Source: CAD feature listing. Evaluate the final solid. Frame: model axes, mm. A direction names the side the tool comes from. Coordinates: 2 decimals unless noted, no trailing zeros. Write each loop counter-clockwise with the first axis right and the second up, starting at its lowest first coordinate (ties: lowest second). Pieces come first, ordered by that corner, then holes. Notation, with made-up numbers: M 4.5,-22.75 L 43.5,-22.75 A16 cw 43.5,-18.75 Z; hole C -14,-15 d5. An arc over 180 degrees is marked long. Answer as CSV lines item,"result". Start each with the question number.
1. Mould query, pull axis Z, two halves, no side actions, for faces 1 (the face through (20, 2, 33.39)), 2 (the face through (37, 2, 63.14)), 3 (the face through (58.326, 2, 27)). Classes: pulls with the +Z half, pulls with the -Z half, needs draft (parallel to the pull), parting line crosses it, or undercut.
2. Section A-A on x = 21. Return the cut outline in (y, z), plus the area to 3 significant figures.
3. Line query: probe 1 along Z at (x, y) = (20, 0.65); probe 2 along X at (y, z) = (0.45, 46.5); probe 3 along Z at (x, y) = (35, 3.5). Output: solid intervals per line, ascending. Write a range as [from, to].
4. Contact query for a flat-ended pin moving along its axis: pin 1 Ø1.2 at (y, z) = (2.5, 45.5) entering from -X. Output: stop coordinate, or through.
5. Section B-B on z = 41. Return the cut outline in (x, y), plus the area to 3 significant figures.
6. Section C-C on y = 2.45. Return the cut outline in (x, z), plus the area to 3 significant figures.
7. Reachability of faces 4 (the face through (58.326, 2, 57)), 5 (the face through (24.326, 2, 42)), 6 (the face through (54, 2, 50.39)) from +Z, -Z, +X, -X, +Y, -Y: full face, straight path, thin tool, end or side. Return the list, or none.
```python
from build123d import *

# Parameters (mm, degrees)
SKETCH_1_W          = 43
SKETCH_1_H          = 42.5
SKETCH_1_R          = 3.2
EXTRUDE_1_DEPTH     = 4
SKETCH_2_W          = 9
SKETCH_2_H          = 17
CUT_EXTRUDE_1_DEPTH = 4


with BuildPart() as part:
    # Эскиз1 → Бобышка-Вытянуть1 (new body)
    with BuildSketch(Plane(origin=(0, 0, 0), x_dir=(1, 0, 0), z_dir=(0, 1, 0))):
        with Locations((36.826052882, -41.88992321)):
            Rectangle(SKETCH_1_W, SKETCH_1_H)
        with Locations(Location((36.826052882, -41.88992321, 0), (0, 0, 270))):
            Circle(SKETCH_1_R, mode=Mode.SUBTRACT)
    extrude(amount=EXTRUDE_1_DEPTH)

    # Эскиз2 → Вырез-Вытянуть1 (cut)
    with BuildSketch(Plane(origin=(0, 4, 0), x_dir=(1, 0, 0), z_dir=(0, 1, 0))):
        with Locations((19.826052882, -41.88992321)):
            Rectangle(SKETCH_2_W, SKETCH_2_H)
        with Locations((53.826052882, -41.88992321)):
            Rectangle(SKETCH_2_W, SKETCH_2_H)
    extrude(amount=-CUT_EXTRUDE_1_DEPTH, mode=Mode.SUBTRACT)


solid = part.part
```
Values:
1,face 1,"undercut"
1,face 2,"pulls with the +Z half"
1,face 3,"needs draft"
2,outline,"M 0,20.64 L 4,20.64 L 4,33.39 L 0,33.39 Z; M 0,50.39 L 4,50.39 L 4,63.14 L 0,63.14 Z"
2,area,"102 mm²"
3,probe 1,"[20.64, 33.39], [50.39, 63.14]"
3,probe 2,"[24.33, 49.33]"
3,probe 3,"[20.64, 39.26], [44.52, 63.14]"
4,pin 1,"x = 24.33"
5,outline,"M 24.33,0 L 33.75,0 L 33.75,4 L 24.33,4 Z; M 39.9,0 L 49.33,0 L 49.33,4 L 39.9,4 Z"
5,area,"75.4 mm²"
6,outline,"M 15.33,20.64 L 58.33,20.64 L 58.33,33.39 L 49.33,33.39 L 49.33,50.39 L 58.33,50.39 L 58.33,63.14 L 15.33,63.14 L 15.33,50.39 L 24.33,50.39 L 24.33,33.39 L 15.33,33.39 Z; hole C 36.83,41.89 d6.4"
6,area,"1,490 mm²"
7,face 4,"+Z, -Z, +X, +Y, -Y"
7,face 5,"-X, +Y, -Y"
7,face 6,"+X, +Y, -Y"
